```python
from build123d import *

# Parameters (mm, degrees)
F0_R          = 45.9121697242
F1_DEPTH      = 42.164
F2_W          = 74.4279101491
F2_H          = 17.0120932162
F3_DEPTH      = 114.3
F5_DEPTH      = 5.08
F5_DEPTH_BACK = 5.08
F6_R          = 24.8732317419
F7_DEPTH      = 42.165


with BuildPart() as f1:
    # F0 (on Top) → F1 (new body)
    with BuildSketch(Plane.XY):
        Circle(F0_R)
    extrude(amount=F1_DEPTH)

    # F2 (on Right) → F3 (join)
    with BuildSketch(Plane.YZ):
        with Locations((0.265814364, 8.5060466081)):
            Rectangle(F2_W, F2_H)
    extrude(amount=F3_DEPTH)

    # F4 (on Front) → F5 (join, two sides)
    with BuildSketch(Plane.XZ) as f5_sk:
        Polygon((42.707439512, 17.0120932162), (100.3890708089, 17.0120932162), (42.707439512, 40.9353487194), align=None)
    extrude(amount=F5_DEPTH)
    extrude(f5_sk.sketch, amount=-F5_DEPTH_BACK)

    # F6 (on face) → F7 (cut, through all)
    with BuildSketch(Plane.XY.offset(42.164)):
        Circle(F6_R)
    extrude(amount=-F7_DEPTH, mode=Mode.SUBTRACT)


solid = f1.part
```
Geometry: final body of the model. Coordinates: model frame, mm. A direction names the side the tool comes from. Round coordinates to 2 decimals unless told otherwise and drop trailing zeros. Loops run counter-clockwise (first coordinate to the right, second up) from the corner with the lowest first, then second, coordinate; pieces in that order, holes last. Notation, with made-up numbers: (65, 44) -> (98, 44) arc R19 cw to (98, 58) -> close; hole circle Ø7 at (55, 14.5). An arc over 180 degrees is marked (long way). Use one line per item in the form item = value.
Item 1: Cut plane B-B on y = 23. Output: boundary loops of the cut face in (x, z).
Evaluation:
outline = (-39.74, 0) -> (-9.47, 0) -> (-9.47, 42.16) -> (-39.74, 42.16) -> close; (9.47, 0) -> (114.3, 0) -> (114.3, 17.01) -> (39.74, 17.01) -> (39.74, 42.16) -> (9.47, 42.16) -> close
Item 2: Cut plane A-A on x = 0. Output: boundary loops of the cut face in (y, z), then the cut area to 3 significant figures.
Evaluation:
outline = (-45.91, 0) -> (-24.87, 0) -> (-24.87, 42.16) -> (-45.91, 42.16) -> close; (24.87, 0) -> (45.91, 0) -> (45.91, 42.16) -> (24.87, 42.16) -> close
area = 1,770 mm2
Item 3: Contact query for flat-ended pins moving along their axis: pin 1 Ø12 at (y, z) = (-1.5, 30.5) entering from +X; pin 2 Ø10 at (x, y) = (96, -32) entering from +Z; pin 3 Ø4 at (x, z) = (63.5, 36) entering from -Y; pin 4 Ø5 at (y, z) = (3.5, 36) entering from -X. Output: stop coordinate, or through.
Evaluation:
pin_1 = 82.33
pin_2 = 17.01
pin_3 = through
pin_4 = -45.9
Item 4: Material intervals for probe 1 along Y at (x, z) = (0, 13); probe 2 along X at (y, z) = (-2, 32); probe 3 along Y at (x, z) = (-15.5, 29.5), sorted ascending.
Evaluation:
probe_1 = -45.91 to -24.87, 24.87 to 45.91
probe_2 = -45.87 to -24.79, 24.79 to 64.25
probe_3 = -43.22 to -19.45, 19.45 to 43.22
Item 5: Draft query along X for faces 6 (the cylindrical face through (-19.74, -15.13, 21.38)), 7 (the flat face through (70, 37.48, 8)), 8 (the flat face through (73.39, -0.07, 28.21)). Return one class per face: released by +X, released by -X, zero draft, split by the parting line, or undercut.
Evaluation:
face_6 = undercut
face_7 = zero draft
face_8 = released by +X
Item 6: Cut plane C-C on x = 37.5. Output: boundary loops of the cut face in (y, z), then the cut area to 3 significant figures.
Evaluation:
outline = (-36.95, 0) -> (37.48, 0) -> (37.48, 17.01) -> (26.49, 17.01) -> (26.49, 42.16) -> (-26.49, 42.16) -> (-26.49, 17.01) -> (-36.95, 17.01) -> close
area = 2,600 mm2
Item 7: Cut plane D-D on y = 0. Output: boundary loops of the cut face in (x, z).
Evaluation:
outline = (-45.91, 0) -> (-24.87, 0) -> (-24.87, 42.16) -> (-45.91, 42.16) -> close; (24.87, 0) -> (114.3, 0) -> (114.3, 17.01) -> (100.39, 17.01) -> (45.91, 39.61) -> (45.91, 42.16) -> (24.87, 42.16) -> close
Item 8: Access query for faces 1 (the flat face through (70, -36.948, 8)), 2 (the cylindrical face through (-45.868, 2.019, 20.787)), 3 (the flat face through (60, 5.08, 23)), 4 (the flat face through (60, -5.08, 23)), 5 (the flat face through (80, 8, 17.012)). Directions: +Z, -Z, +X, -X, +Y, -Y. A direction counts if a zero-diameter tool reaches every point of the face in a straight line with its end or side. Return the directions, or none.
Evaluation:
face_1 = +Z, -Z, +X, -Y
face_2 = +Z
face_3 = +Z, +X, +Y
face_4 = +Z, +X, -Y
face_5 = +Z, +X
